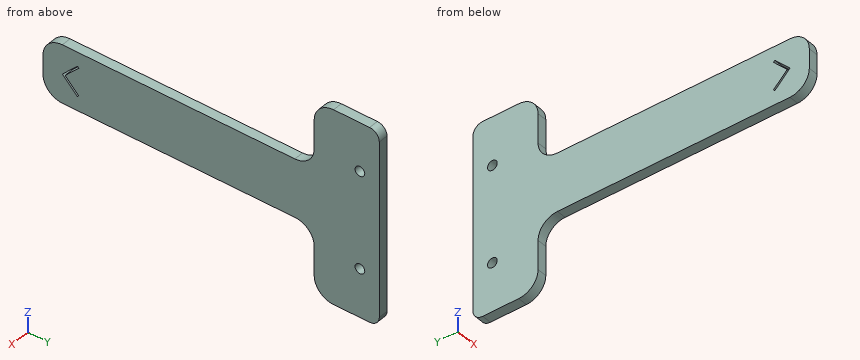
from build123d import *

# Parameters (mm, degrees)
BOSS_EXTRUDE2_DEPTH     = 6.35
CUT_EXTRUDE1_REACH      = 129.376
CUT_EXTRUDE2_DEPTH      = 128.37561853
CUT_EXTRUDE2_DEPTH_BACK = 128.37561853
SKETCH5_R               = 3.175
CUT_EXTRUDE3_DEPTH      = 128.37561853


with BuildPart() as part:
    # Sketch3 → Boss-Extrude2 (new body)
    with BuildSketch(Plane(origin=(0, 0, 0), x_dir=(0, 0, -1), z_dir=(1, 0, 0))):
        with BuildLine():
            Line((-57.15, -110.236), (57.15, -110.236))
            ThreePointArc((57.15, -110.236), (61.640128061, -108.376128061), (63.5, -103.886))
            Line((63.5, -103.886), (63.5, 103.886))
            ThreePointArc((63.5, 103.886), (61.640128061, 108.376128061), (57.15, 110.236))
            Line((57.15, 110.236), (-57.15, 110.236))
            ThreePointArc((-57.15, 110.236), (-61.640128061, 108.376128061), (-63.5, 103.886))
            Line((-63.5, 103.886), (-63.5, -103.886))
            ThreePointArc((-63.5, -103.886), (-61.640128061, -108.376128061), (-57.15, -110.236))
        make_face()
    extrude(amount=BOSS_EXTRUDE2_DEPTH)

    # Sketch4 → Cut-Extrude1 (cut, up to next)
    with BuildSketch(Plane(origin=(6.35, 0, 0), x_dir=(0, 0, -1), z_dir=(1, 0, 0)), mode=Mode.PRIVATE) as cut_extrude1_sk1:
        Polygon((0, -95.739948776), (-8.980256121, -86.759692655), (-9.878281733, -87.657718267), (0, -97.536), (9.878281733, -87.657718267), (8.980256121, -86.759692655), align=None)
    cut_extrude1_tool1 = extrude(cut_extrude1_sk1.sketch, amount=-CUT_EXTRUDE1_REACH, mode=Mode.PRIVATE) & part.part
    add(cut_extrude1_tool1.solids().sort_by_distance((6.35, -91.408951, 4.649259))[0], mode=Mode.SUBTRACT)

    # Sketch5 → Cut-Extrude2 (cut, two sides: drawn at the far end of the back side and taken through both)
    with BuildSketch(Plane(origin=(6.35, 0, 0), x_dir=(0, 0, -1), z_dir=(1, 0, 0)).offset(-CUT_EXTRUDE2_DEPTH_BACK)):
        with Locations((-31.75, 97.536)):
            Circle(SKETCH5_R)
        with Locations((31.75, 97.536)):
            Circle(SKETCH5_R)
    extrude(amount=CUT_EXTRUDE2_DEPTH + CUT_EXTRUDE2_DEPTH_BACK, mode=Mode.SUBTRACT)

    # Sketch6 → Cut-Extrude3 (cut, through all)
    with BuildSketch(Plane(origin=(6.35, 0, 0), x_dir=(0, 0, -1), z_dir=(1, 0, 0))):
        with BuildLine():
            Line((-19.05, -97.536), (-19.05, 54.864))
            ThreePointArc((-19.05, 54.864), (-22.769743879, 63.844256121), (-31.75, 67.564))
            Line((-31.75, 67.564), (-50.8, 67.564))
            ThreePointArc((-50.8, 67.564), (-59.780256121, 71.283743879), (-63.5, 80.264))
            Line((-63.5, 80.264), (-63.5, 67.564))
            Line((-63.5, 67.564), (-63.5, -103.886))
            ThreePointArc((-63.5, -103.886), (-61.640128061, -108.376128061), (-57.15, -110.236))
            Line((-57.15, -110.236), (-19.05, -110.236))
            Line((-19.05, -110.236), (-6.35, -110.236))
            ThreePointArc((-6.35, -110.236), (-15.330256121, -106.516256121), (-19.05, -97.536))
        make_face()
        with BuildLine():
            Line((19.05, -97.536), (19.05, 54.864))
            ThreePointArc((19.05, 54.864), (22.769743879, 63.844256121), (31.75, 67.564))
            Line((31.75, 67.564), (50.8, 67.564))
            ThreePointArc((50.8, 67.564), (59.780256121, 71.283743879), (63.5, 80.264))
            Line((63.5, 80.264), (63.5, 67.564))
            Line((63.5, 67.564), (63.5, -103.886))
            ThreePointArc((63.5, -103.886), (61.640128061, -108.376128061), (57.15, -110.236))
            Line((57.15, -110.236), (19.05, -110.236))
            Line((19.05, -110.236), (6.35, -110.236))
            ThreePointArc((6.35, -110.236), (15.330256121, -106.516256121), (19.05, -97.536))
        make_face()
    extrude(amount=-CUT_EXTRUDE3_DEPTH, mode=Mode.SUBTRACT)


solid = part.part
Can you work these out from the model? Positions are in its coordinate system, mm. Coordinates: 2 decimals unless noted, no trailing zeros. Write each loop counter-clockwise with the first axis right and the second up, starting at its lowest first coordinate (ties: lowest second). Pieces come first, ordered by that corner, then holes. Notation, with made-up numbers: (-24, 6.5) - (-17, 6.5) arc R28 cw to (-17, 25.5) - close; hole circle Ø6 at (61.25, 57). An arc over 180 degrees is marked (long way). Return JSON: item names as keys, results as strings. Group by question number.
Item 1: I'm going to push flat-ended pins straight in: pin 1 Ø3 at (x, y) = (4, -22.5) entering from +Z; pin 2 Ø3 at (x, z) = (4, -38.5) entering from -Y; pin 3 Ø1 at (x, z) = (1, 25) entering from -Y. Where does each tip first touch, or does it pass through?
Item 2: If we section it at A-A (x = 2.75): Write out the boundary of the cut face in (y, z) (3 decimals).
Item 3: If we section it at C-C (y = -82): Write out the boundary of the cut face in (x, z), then the cut area to 3 significant figures.
Item 4: Please list where these lines run through material, in increasing order: probe 1 along Y at (x, z) = (3.5, -31.75); probe 2 along Z at (x, y) = (2, -0.5); probe 3 along Y at (x, z) = (3, 41).
Item 5: If we section it at B-B (z = -54.5): Write out the boundary of the cut face in (x, y).
Return value:
{
 "1": {"pin 1": "stops at z = 19.05", "pin 2": "stops at y = 67.56", "pin 3": "stops at y = 65.29"},
 "2": {"outline": "(-110.236, -6.35) arc R12.7 ccw to (-97.536, -19.05) - (54.864, -19.05) arc R12.7 cw to (67.564, -31.75) - (67.564, -50.8) arc R12.7 ccw to (80.264, -63.5) - (103.886, -63.5) arc R6.35 ccw to (110.236, -57.15) - (110.236, 57.15) arc R6.35 ccw to (103.886, 63.5) - (80.264, 63.5) arc R12.7 ccw to (67.564, 50.8) - (67.564, 31.75) arc R12.7 cw to (54.864, 19.05) - (-97.536, 19.05) arc R12.7 ccw to (-110.236, 6.35) - close; hole (-97.536, 0) - (-87.658, -9.878) - (-86.76, -8.98) - (-95.74, 0) - (-86.76, 8.98) - (-87.658, 9.878) - close; hole circle Ø6.35 at (97.536, -31.75); hole circle Ø6.35 at (97.536, 31.75)"},
 "3": {"outline": "(0, -19.05) - (6.35, -19.05) - (6.35, 19.05) - (0, 19.05) - close", "area": "242 mm^2"},
 "4": {"probe 1": "y = 67.56 to 94.36, 100.71 to 110.24", "probe 2": "z = -19.05 to 19.05", "probe 3": "y = 67.56 to 110.24"},
 "5": {"outline": "(0, 68.11) - (6.35, 68.11) - (6.35, 110.24) - (0, 110.24) - close"}
}
